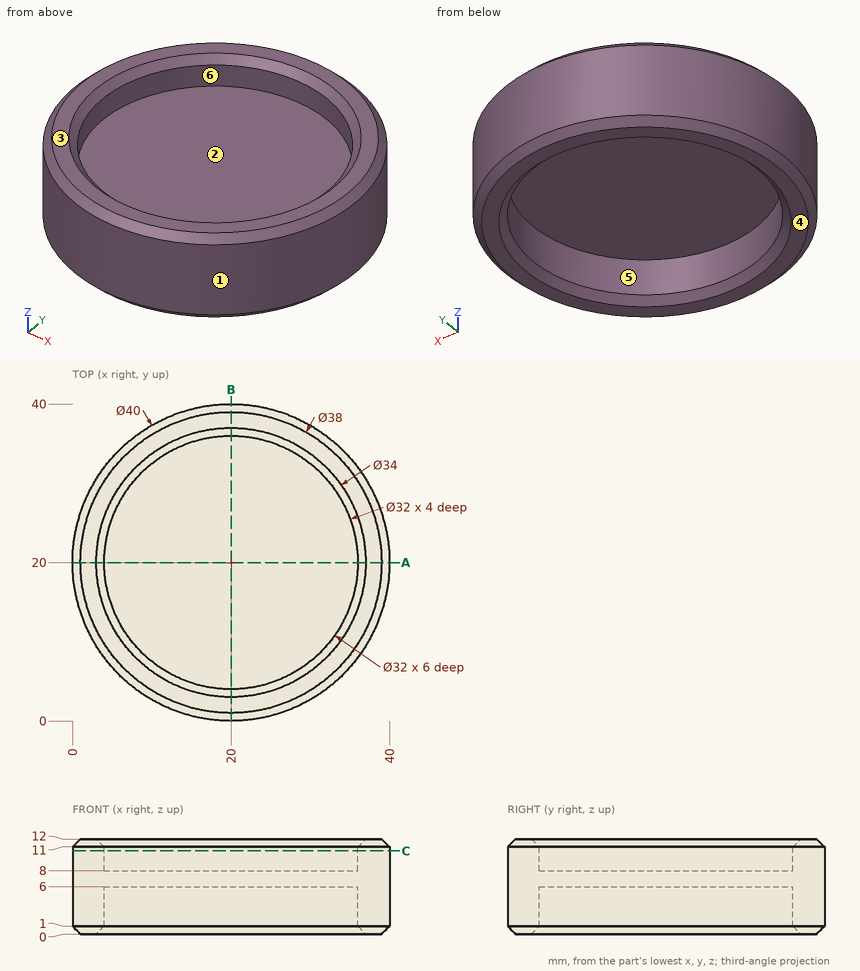
Check sheet for the drawn part. Datum: minimum x, y, z corner. Units: mm. A direction names the side the tool comes from. Round coordinates to 2 decimals unless told otherwise and drop trailing zeros. Order: outer loops, then holes, each group sorted by start corner. A loop starts at its lowest first (then second) coordinate and runs counter-clockwise, first axis right, second up.
1. Section check A-A on y = 20. Record the cut outline in (x, z).
Final values:
outline: (0, 1) - (1, 0) - (3, 0) - (4, 1) - (4, 6) - (36, 6) - (36, 1) - (37, 0) - (39, 0) - (40, 1) - (40, 11) - (39, 12) - (37, 12) - (36, 11) - (36, 8) - (4, 8) - (4, 11) - (3, 12) - (1, 12) - (0, 11) - close
2. Section check C-C on z = 10.5. Record the cut outline in (x, y).
Final values:
outline: circle Ø40 at (20, 20); hole circle Ø32 at (20, 20)
3. Thickness scan on L1, parallel to Y at x = 20, z = 10; L2, parallel to Z at x = 27, y = 30. Record the ranges inside material, lowest first.
Final values:
L1: y = 0 to 4, 36 to 40
L2: z = 6 to 8
4. Access from +Z, -Z, +X, -X, +Y, -Y to the whole of each face (thin tool, end or side, straight path). Record for the marked faces 4, 5 and 6.
Final values:
face 4: -Z, +X, -X, +Y, -Y
face 5: -Z
face 6: +Z
5. Go/stop test with flat-tipped pins: P1, Ø2, axis at x = 6.5, y = 28.5, coming from the -Z side; P2, Ø12, axis at x = 34, y = 6.5, coming from the +Z side; P3, Ø9.5, axis at x = 13, y = 19.5, coming from the +Z side; P4, Ø2, axis at x = 24, z = 5, coming from the -Y side. Record where each tip stops, or that it passes through.
Final values:
P1: stops at z = 0.05
P2: stops at z = 12
P3: stops at z = 8
P4: stops at y = 0.23
6. Release check for a two-part mould opening along Y. For the marked faces 1, 2 and 3 record: +Y half, -Y half, draft (parallel to the pull), parting line (faces both ways), or undercut.
Final values:
face 1: parting line
face 2: undercut
face 3: draft
